from build123d import *

# Parameters (mm, degrees)
EXTRUDE_1_DEPTH     = 50
CUT_EXTRUDE_START   = -19.5
SKETCH_2_R          = 1.5
CUT_EXTRUDE_1_DEPTH = 70
SKETCH_3_OUTSIDE_W  = 61.218
SKETCH_3_OUTSIDE_H  = 66.218
CUT_EXTRUDE_2_DEPTH = 70
SKETCH_2_3_R        = 1.5
CUT_EXTRUDE_4_DEPTH = 10
SKETCH_5_R          = 1
CUT_EXTRUDE_5_DEPTH = 10
FILLET_1_R          = 5
SKETCH_6_W          = 13
SKETCH_6_H          = 23.5
CUT_EXTRUDE_6_DEPTH = 10
SKETCH_7_R          = 1.65
CUT_EXTRUDE_7_DEPTH = 10


with BuildPart() as part:
    # Sketch 1 → Extrude 1 (new body)
    with BuildSketch(Plane.XY):
        Polygon((-45, 11.5), (0, 11.5), (0, -11.5), (-45, -11.5), (-45, -8), (-3.5, -8), (-3.5, 8), (-45, 8), align=None)
    extrude(amount=EXTRUDE_1_DEPTH)

    # Sketch 2 → Cut-Extrude 1 (cut)
    with BuildSketch(Plane.XZ.offset(11.5).offset(CUT_EXTRUDE_START)):
        with Locations((-16, 35)):
            Circle(SKETCH_2_R)
        with Locations((-16, 15)):
            Circle(SKETCH_2_R)
        with Locations((-31, 30)):
            Circle(SKETCH_2_R)
        with Locations((-31, 20)):
            Circle(SKETCH_2_R)
    extrude(amount=-CUT_EXTRUDE_1_DEPTH, mode=Mode.SUBTRACT)

    # Sketch 3 outside → Cut-Extrude 2 (cut)
    with BuildSketch(Plane.XZ.offset(11.5)):
        with Locations((-22.5, 25)):
            Rectangle(SKETCH_3_OUTSIDE_W, SKETCH_3_OUTSIDE_H)
        Polygon((-21, 0), (-36, 15), (-36, 35), (-21, 50), (0, 50), (0, 0), align=None, mode=Mode.SUBTRACT)
    extrude(amount=-CUT_EXTRUDE_2_DEPTH, mode=Mode.SUBTRACT)

    # Sketch 2_3 → Cut-Extrude 4 (cut)
    with BuildSketch(Plane.XZ.offset(11.5)):
        with Locations((-31, 30)):
            Circle(SKETCH_2_3_R)
        with Locations((-31, 20)):
            Circle(SKETCH_2_3_R)
    extrude(amount=-CUT_EXTRUDE_4_DEPTH, mode=Mode.SUBTRACT)

    # Sketch 5 → Cut-Extrude 5 (cut)
    with BuildSketch(Plane.XZ.offset(11.5)):
        with Locations((-16, 43.045)):
            Circle(SKETCH_5_R)
        with Locations((-16, 15.375)):
            Circle(SKETCH_5_R)
    extrude(amount=-CUT_EXTRUDE_5_DEPTH, mode=Mode.SUBTRACT)

    # Fillet 1
    fillet_1_edges = [part.edges().sort_by_distance(p)[0] for p in [
        (-21, -9.75, 0),
        (-21, 9.75, 0),
        (-21, -9.75, 50),
        (-21, 9.75, 50),
        (-36, 9.75, 35),
        (-36, -9.75, 35),
        (-36, 9.75, 15),
        (-36, -9.75, 15),
    ]]
    fillet(fillet_1_edges, radius=FILLET_1_R)

    # Sketch 6 → Cut-Extrude 6 (cut)
    with BuildSketch(Plane.XZ.offset(11.5)):
        with Locations((-16, 29.21)):
            Rectangle(SKETCH_6_W, SKETCH_6_H)
    extrude(amount=-CUT_EXTRUDE_6_DEPTH, mode=Mode.SUBTRACT)

    # Sketch 7 → Cut-Extrude 7 (cut)
    with BuildSketch(Plane(origin=(0, 0, 0), x_dir=(0, 0, -1), z_dir=(1, 0, 0))):
        with Locations((-10, 0)):
            Circle(SKETCH_7_R)
        with Locations((-40, 0)):
            Circle(SKETCH_7_R)
    extrude(amount=-CUT_EXTRUDE_7_DEPTH, mode=Mode.SUBTRACT)


solid = part.part
Geometry: final body of the model. Coordinates: model frame, mm. A direction names the side the tool comes from. Give positions to 0.01 mm unless a question says otherwise; leave off trailing zeros. Loops run counter-clockwise (first coordinate to the right, second up) from the corner with the lowest first, then second, coordinate; pieces in that order, holes last. Notation, with made-up numbers: M 83,47.5 L 102,47.5 A26 ccw 102,74.5 Z; hole C 15,13 d11. An arc over 180 degrees is marked long. Put each result on its own line as item: value.
1) Cut plane C-C, the plane z = 20. Return the cut outline in (x, y), plus the area to 4 significant figures.
Computed values:
outline: M -36,-11.5 L -32.5,-11.5 L -32.5,-8 L -36,-8 Z; M -36,8 L -32.5,8 L -32.5,11.5 L -36,11.5 Z; M -29.5,-11.5 L -22.5,-11.5 L -22.5,-8 L -29.5,-8 Z; M -29.5,8 L -3.5,8 L -3.5,-8 L -9.5,-8 L -9.5,-11.5 L 0,-11.5 L 0,11.5 L -29.5,11.5 Z
area: 241.5 mm^2
2) Cut plane B-B, the plane x = -31. Return the cut outline in (y, z).
Computed values:
outline: M -11.5,10 L -8,10 L -8,18.5 L -11.5,18.5 Z; M -11.5,21.5 L -8,21.5 L -8,28.5 L -11.5,28.5 Z; M -11.5,31.5 L -8,31.5 L -8,40 L -11.5,40 Z; M 8,10 L 11.5,10 L 11.5,18.5 L 8,18.5 Z; M 8,21.5 L 11.5,21.5 L 11.5,28.5 L 8,28.5 Z; M 8,31.5 L 11.5,31.5 L 11.5,40 L 8,40 Z
3) First-contact query: P1, Ø2, axis at y = 0, z = 40, coming from the -X side; P2, Ø4, axis at y = 0, z = 10, coming from the -X side; P3, Ø5, axis at x = -16, z = 35, coming from the -Y side. Flat tips, straight axial feed; report the tip coordinate or a pass-through.
Computed values:
P1: passes through
P2: stops at x = -3.5
P3: stops at y = 8
4) Cut plane A-A, the plane z = 10. Return the cut outline in (x, y), plus the area to 3 significant figures.
Computed values:
outline: M -31,-11.5 L 0,-11.5 L 0,-1.65 L -3.5,-1.65 L -3.5,-8 L -31,-8 Z; M -31,8 L -3.5,8 L -3.5,1.65 L 0,1.65 L 0,11.5 L -31,11.5 Z
area: 261 mm^2
5) Reachability of faces 1 (the flat face through (-22.5, -10, 29)), 2 (the flat face through (-3.5, 0, 25)), 3 (the flat face through (0, 0, 25)) from +Z, -Z, +X, -X, +Y, -Y: full face, straight path, thin tool, end or side. Return the list, or none.
Computed values:
face 1: -Y
face 2: +Z, -Z, -X
face 3: +Z, -Z, +X, +Y, -Y
6) Cut plane D-D, the plane y = 0. Return the cut outline in (x, z).
Computed values:
outline: M -3.5,0 L 0,0 L 0,8.35 L -3.5,8.35 Z; M -3.5,11.65 L 0,11.65 L 0,38.35 L -3.5,38.35 Z; M -3.5,41.65 L 0,41.65 L 0,50 L -3.5,50 Z
7) Mould query, pull axis Z, two halves, no side actions, for faces 4 (the cylindrical face through (-20.82, 9.77, 0.37)), 5 (the flat face through (-29, 10, 42)), 6 (the cylindrical face through (-1.726, -0.632, 8.476)), 7 (the cylindrical face through (-15.539, -9.774, 14.488)). Classes: released by +Z, released by -Z, zero draft, split by the parting line, or undercut.
Computed values:
face 4: released by -Z
face 5: released by +Z
face 6: undercut
face 7: undercut
8) Material intervals for L1, parallel to Y at x = -8, z = 33.5; L2, parallel to X at y = -1.5, z = 42.5; L3, parallel to Y at x = -2, z = 40, sorted ascending. Write a range as from..to.
Computed values:
L1: y = -11.5..-8, 8..11.5
L2: x = -3.5..0
L3: y = -11.5..-1.65, 1.65..11.5
